Design review of the part built by this model. Coordinates are the model's own, in mm. A direction names the side the tool comes from. Coordinates: 2 decimals unless noted, no trailing zeros. Loops run counter-clockwise (first coordinate to the right, second up) from the corner with the lowest first, then second, coordinate; pieces in that order, holes last. Notation, with made-up numbers: M 84.5,51.5 L 139.5,51.5 A4 cw 139.5,56.5 Z; hole C 54.5,77 d10. An arc over 180 degrees is marked long. Write item = value, one per line. Start each with the question number.
Autodesk Fusion 360 part; units mm, degrees
sketch "Sketch1" plane through (0, 0, 0) normal (0, 0, 1) x (1, 0, 0)
  line L0 (0, 0) -> (19.25, 0)
  line L1 (19.25, 0) -> (19.25, -3)
  line L2 (19.25, -3) -> (19.25, -5.7)
  line L3 (19.25, -5.7) -> (19.25, -12.3)
  line L4 (19.25, -12.3) -> (17.25, -12.3)
  line L5 (17.25, -12.3) -> (17.25, -0.6)
  line L6 (19.25, -3) -> (19.25, -4.35) construction
  line L7 (19.25, -4.35) -> (18.75, -4.35) construction
  line L8 (19.25, -3) -> (18.75, -4.35)
  line L9 (18.75, -4.35) -> (19.25, -5.7)
  line L10 (0, 0) -> (0, -0.6)
  line L11 (0, -0.6) -> (17.25, -0.6)
  dimension "d1" = 19.25
  dimension "d2" = 3
  dimension "d4" = 2.7
  dimension "d5" = 6.6
  dimension "d6" = 2
  dimension "d7" = 11.7
  dimension "d8" = 1.35
  dimension "d9" = 0.5
  dimension "d10" = 17.25
  dimension "d11" = 0.6
  dimension "d12" = 19.25
revolve "Revolve1" add sketch "Sketch1" angle 360 about axis through (0, 0, 0) along (0, -1, 0) contours L0 L1 L3 L4 L5 L8 L9 L10 L11
sketch "Sketch2" plane through (0, 0, 0) normal (0, 1, 0) x (-1, 0, 0)
  circle A0 centre (0, 0) radius 19.25
  circle A1 centre (0, 0) radius 18.825
  circle A2 centre (0, 0) radius 4.7
  dimension "d14" = 38.5
  dimension "d15" = 37.65
  dimension "d16" = 9.4
extrude "Extrude1" cut sketch "Sketch2" against normal blind 3 contours A2
equation "d15 = d14 - 0.85 mm"
Q1. Clearance check with flat-ended pins moving along their axes: P1, Ø1, axis at y = -2.5, z = 0.5, coming from the -X side; P2, Ø11, axis at x = 0, z = 0, coming from the -Y side; P3, Ø5, axis at x = 14.5, y = -10, coming from the +Z side; P4, Ø2, axis at x = -6.5, y = -1.5, coming from the +Z side. State where each tip first meets the part, or that it passes through.
Q2. Add section B-B on z = 0. State the section outline as (x, y) points.
Q3. Add section A-A on x = 0. State the section outline as (y, z) points.
Q4. For faces 4 (the face through (16.453, -6.368, -5.181)), 5 (the face through (-15.28, -1.52, -11.71)), list the 3-axis set-ups (+Z, -Z, +X, -X, +Y, -Y) from which the entire face can be reached by the end or side of a thin tool; tool diameter is ignored.
Q5. Mouldability with a two-part tool opening along Z and no side actions: class faces 1 (the face through (4, -0.6, -4)), 2 (the face through (-15.28, -9.05, -11.71)), 3 (the face through (4, 0, -4)) as released by +Z, released by -Z, zero draft, split by the parting line, or undercut.
Q6. To check wall thickness, follow line 1 (Z direction, x = 0, y = -0.15); line 2 (Z direction, x = 0, y = -11.5); line 3 (Y direction, x = 6.5, z = 11). State the ranges of each line that lie inside material, in increasing order. Write a range as from..to.
Q7. Add section C-C on y = -2. State the section outline as (x, z) points, plus the area to 3 significant figures.
Values follow:
q1.P1 = -19.25
q1.P2 = -0.6
q1.P3 = 15.05
q1.P4 = 18.45
q2.outline = M -19.25,-12.3 L -17.25,-12.3 L -17.25,-0.6 L -4.7,-0.6 L -4.7,0 L -19.25,0 L -19.25,-3 L -18.75,-4.35 L -19.25,-5.7 Z; M 4.7,-0.6 L 17.25,-0.6 L 17.25,-12.3 L 19.25,-12.3 L 19.25,-5.7 L 18.75,-4.35 L 19.25,-3 L 19.25,0 L 4.7,0 Z
q3.outline = M -12.3,-19.25 L -5.7,-19.25 L -4.35,-18.75 L -3,-19.25 L 0,-19.25 L 0,-4.7 L -0.6,-4.7 L -0.6,-17.25 L -12.3,-17.25 Z; M -12.3,17.25 L -0.6,17.25 L -0.6,4.7 L 0,4.7 L 0,19.25 L -3,19.25 L -4.35,18.75 L -5.7,19.25 L -12.3,19.25 Z
q4.face_4 = -Y
q4.face_5 = +Y, -Y
q5.face_1 = undercut
q5.face_2 = split by the parting line
q5.face_3 = zero draft
q6.line_1 = -19.25..-4.7, 4.7..19.25
q6.line_2 = -19.25..-17.25, 17.25..19.25
q6.line_3 = -0.6..0
q7.outline = C 0,0 d38.5; hole C 0,0 d34.5
q7.area = 229 mm2
